```python
from build123d import *

# Parameters (mm, degrees)
SKIZZE1_R                       = 11.5
AUFSATZ_LINEAR_AUSTRAGEN1_DEPTH = 77
SKIZZE2_R                       = 7.1
SCHNITT_LINEAR_AUSTRAGEN1_DEPTH = 4.1
SKIZZE3_R                       = 2.1
SCHNITT_LINEAR_AUSTRAGEN2_DEPTH = 3
SKIZZE4_R                       = 9.6
SCHNITT_LINEAR_AUSTRAGEN3_DEPTH = 12.75
SCHNITT_LINEAR_START            = -6
SKIZZE7_W                       = 1.5
SKIZZE7_H                       = 15
SCHNITT_LINEAR_AUSTRAGEN4_DEPTH = 63
SKIZZE8_W                       = 63
SKIZZE8_H                       = 4
AUFSATZ_LINEAR_AUSTRAGEN2_DEPTH = 1.5
SCHNITT_LINEAR_AUSTRAGEN6_DEPTH = 13.5
SKIZZE12_R                      = 3
SCHNITT_LINEAR_AUSTRAGEN7_DEPTH = 2
KREISMUSTER3_COUNT              = 3
SKIZZE13_R                      = 8.5
SCHNITT_LINEAR_AUSTRAGEN8_DEPTH = 40


with BuildPart() as part:
    # Skizze1 → Aufsatz-Linear austragen1 (new body)
    with BuildSketch(Plane(origin=(0, 0, 0), x_dir=(0, 0, -1), z_dir=(1, 0, 0))):
        Circle(SKIZZE1_R)
    extrude(amount=AUFSATZ_LINEAR_AUSTRAGEN1_DEPTH)

    # Skizze2 → Schnitt-Linear austragen1 (cut)
    with BuildSketch(Plane(origin=(77, 0, 0), x_dir=(0, 0, -1), z_dir=(1, 0, 0))):
        Circle(SKIZZE2_R)
    extrude(amount=-SCHNITT_LINEAR_AUSTRAGEN1_DEPTH, mode=Mode.SUBTRACT)

    # Skizze3 → Schnitt-Linear austragen2 (cut)
    with BuildSketch(Plane(origin=(72.9, 0, 0), x_dir=(0, 0, -1), z_dir=(1, 0, 0))):
        Circle(SKIZZE3_R)
    extrude(amount=-SCHNITT_LINEAR_AUSTRAGEN2_DEPTH, mode=Mode.SUBTRACT)

    # Skizze4 → Schnitt-Linear austragen3 (cut)
    with BuildSketch(Plane.ZY):
        Circle(SKIZZE4_R)
    extrude(amount=-SCHNITT_LINEAR_AUSTRAGEN3_DEPTH, mode=Mode.SUBTRACT)

    # Skizze7 → Schnitt-Linear austragen4 (cut)
    with BuildSketch(Plane(origin=(77, 0, 0), x_dir=(0, 0, -1), z_dir=(1, 0, 0)).offset(SCHNITT_LINEAR_START)):
        with Locations((-10.75, 0)):
            Rectangle(SKIZZE7_W, SKIZZE7_H)
    schnitt_linear_austragen4 = extrude(amount=-SCHNITT_LINEAR_AUSTRAGEN4_DEPTH, mode=Mode.SUBTRACT)

    # Skizze8 → Aufsatz-Linear austragen2 (add)
    with BuildSketch(Plane.XY.offset(10)):
        with Locations((39.5, 0)):
            Rectangle(SKIZZE8_W, SKIZZE8_H)
    aufsatz_linear_austragen2 = extrude(amount=AUFSATZ_LINEAR_AUSTRAGEN2_DEPTH)

    # Skizze10 → Schnitt-Linear austragen6 (cut)
    with BuildSketch(Plane.ZY.offset(-12.75)):
        Polygon((4.038863706, -2.240739453), (3.959969143, 2.377388845), (-0.078894563, 4.618128298), (-4.038863706, 2.240739453), (-3.959969143, -2.377388845), (0.078894563, -4.618128298), align=None)
    extrude(amount=-SCHNITT_LINEAR_AUSTRAGEN6_DEPTH, mode=Mode.SUBTRACT)

    # Skizze12 → Schnitt-Linear austragen7 (cut)
    with BuildSketch(Plane.ZY.offset(-26.25)):
        Circle(SKIZZE12_R)
    extrude(amount=-SCHNITT_LINEAR_AUSTRAGEN7_DEPTH, mode=Mode.SUBTRACT)

    # Kreismuster3: Schnitt-Linear austragen4, Aufsatz-Linear austragen2 ×3 about axis
    kreismuster3_axis = Axis((0, 0, 0), (1, 0, 0))
    add([schnitt_linear_austragen4.rotate(kreismuster3_axis, i * 360 / KREISMUSTER3_COUNT) for i in range(1, KREISMUSTER3_COUNT)], mode=Mode.SUBTRACT)
    add([aufsatz_linear_austragen2.rotate(kreismuster3_axis, i * 360 / KREISMUSTER3_COUNT) for i in range(1, KREISMUSTER3_COUNT)])

    # Skizze13 → Schnitt-Linear austragen8 (cut)
    with BuildSketch(Plane(origin=(69.9, 0, 0), x_dir=(0, 0, -1), z_dir=(1, 0, 0))):
        Circle(SKIZZE13_R)
    extrude(amount=-SCHNITT_LINEAR_AUSTRAGEN8_DEPTH, mode=Mode.SUBTRACT)


solid = part.part
```
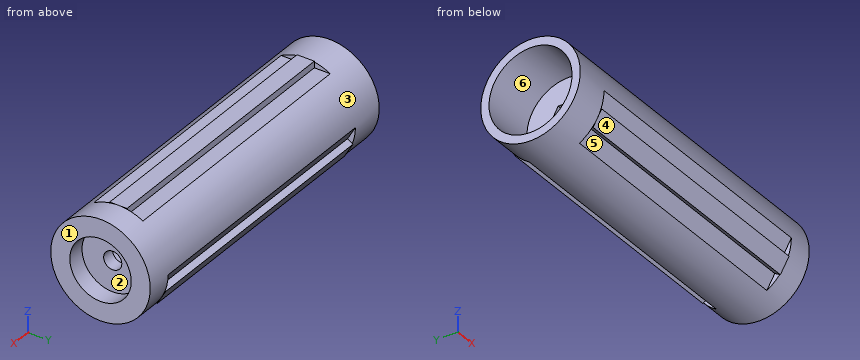
Could you check a few things on this model? Use its own coordinates, in mm. Face numbers are marked on the shaded views. A direction names the side the tool comes from. Coordinates: 2 decimals unless noted, no trailing zeros. Order: outer loops, then holes, each group sorted by start corner. A loop starts at its lowest first (then second) coordinate and runs counter-clockwise, first axis right, second up. Notation, with made-up numbers: M 25.25,83 L 84.25,83 A22 ccw 84.25,113 Z; hole C -22.75,-34 d3. An arc over 180 degrees is marked long. Use a Markdown table: item, result. Add a question column.
Q1. I'm going to push flat-ended pins straight in: pin 1 (9 mm diameter, centred on y = 1.5, z = 1, fed in from -X); pin 2 (1 mm diameter, centred on x = 53.5, z = 7, fed in from +Y); pin 3 (10 mm diameter, centred on x = 45, y = 5.5, fed in from -Z). Where does each tip first touch, or does it pass through?
Q2. If I drill on L1, parallel to X at y = -4.5, z = 3.5; L2, parallel to X at y = -7.5, z = -3; L3, parallel to Y at x = 27.2, z = 0, over which ranges is the centre line in solid material (lowest first)?
Q3. We'd pull the mould along Y, two halves only. Please class the marked faces 1, 2, 3 and 4: pulls with the +Y half, pulls with the -Y half, needs draft (parallel to the pull), parting line crosses it, or undercut.
Q4. I want a section at A-A on x = 38. List the corners of the cut face in (y, z) for me.
Q5. Which directions (+Z, -Z, +X, -X, +Y, -Y) give clear straight access to the entire face, cutting with the end or side of a thin tool? Please do the marked faces 5 and 6.
Q6. I want a section at C-C on x = 15. List the corners of the cut face in (y, z) for me.
Checked values:
| question | item | result |
|---|---|---|
| 1 | pin 1 | x = 12.75 |
| 1 | pin 2 | y = 9.49 |
| 1 | pin 3 | z = -11.49 |
| 2 | L1 | 12.75 to 29.9, 69.9 to 72.9 |
| 2 | L2 | 12.75 to 29.9, 69.9 to 77 |
| 2 | L3 | -11.5 to -3, 3 to 11.5 |
| 3 | face 1 | needs draft |
| 3 | face 2 | undercut |
| 3 | face 3 | parting line crosses it |
| 3 | face 4 | pulls with the -Y half |
| 4 | outline | M -11.5,-0.08 L -9.66,-3.27 L -10.96,-4.02 L -8.96,-7.48 L -7.66,-6.73 L -5.82,-9.92 A11.5 ccw 5.82,-9.92 L 7.66,-6.73 L 8.96,-7.48 L 10.96,-4.02 L 9.66,-3.27 L 11.5,-0.08 A11.5 ccw 5.68,10 L 2,10 L 2,11.5 L -2,11.5 L -2,10 L -5.68,10 A11.5 ccw Z; hole C 0,0 d17 |
| 5 | face 5 | -Z |
| 5 | face 6 | -X |
| 6 | outline | M -11.5,-0.08 L -9.66,-3.27 L -10.96,-4.02 L -8.96,-7.48 L -7.66,-6.73 L -5.82,-9.92 A11.5 ccw 5.82,-9.92 L 7.66,-6.73 L 8.96,-7.48 L 10.96,-4.02 L 9.66,-3.27 L 11.5,-0.08 A11.5 ccw 5.68,10 L 2,10 L 2,11.5 L -2,11.5 L -2,10 L -5.68,10 A11.5 ccw Z; hole M -4.62,0.08 L -2.38,-3.96 L 2.24,-4.04 L 4.62,-0.08 L 2.38,3.96 L -2.24,4.04 Z |
